```python
from build123d import *

# Parameters (mm, degrees)
BOSS_EXTRUDE1_DEPTH = 3
SKETCH2_R           = 1.5
SKETCH2_W           = 14
SKETCH2_H           = 7
CUT_EXTRUDE1_DEPTH  = 3


with BuildPart() as part:
    # Sketch1 → Boss-Extrude1 (new body)
    with BuildSketch(Plane(origin=(0, 0, 0), x_dir=(1, 0, 0), z_dir=(0, 1, 0))):
        Polygon((-41, -41), (-17.5, -41), (-17.5, -38), (17.5, -38), (17.5, -41), (41, -41), (41, -17.5), (38, -17.5), (38, 17.5), (41, 17.5), (41, 41), (17.5, 41), (17.5, 38), (-17.5, 38), (-17.5, 41), (-41, 41), (-41, 17.5), (-38, 17.5), (-38, -17.5), (-41, -17.5), align=None)
    extrude(amount=BOSS_EXTRUDE1_DEPTH)

    # Sketch2 → Cut-Extrude1 (cut)
    with BuildSketch(Plane(origin=(0, 3, 0), x_dir=(1, 0, 0), z_dir=(0, 1, 0))):
        with Locations((0, -8.5)):
            Circle(SKETCH2_R)
        with Locations((0, 13.5)):
            Rectangle(SKETCH2_W, SKETCH2_H)
    extrude(amount=-CUT_EXTRUDE1_DEPTH, mode=Mode.SUBTRACT)


solid = part.part
```
Input: part model. Units: mm. Frame: model coordinates. A direction names the side the tool comes from. Coordinates: 2 decimals unless noted, no trailing zeros. Loops run counter-clockwise (first coordinate to the right, second up) from the corner with the lowest first, then second, coordinate; pieces in that order, holes last.
Q1. Section D-D, the plane z = 8.5. Return the cut outline in (x, y).
Results are:
outline: (-38, 0) - (-1.5, 0) - (-1.5, 3) - (-38, 3) - close; (1.5, 0) - (38, 0) - (38, 3) - (1.5, 3) - close
Q2. Contact query for flat-ended pins moving along their axis: pin 1 (1.5 mm diameter, centred on y = 1, z = -13.5, fed in from +X); pin 2 (0.9 mm diameter, centred on x = -8.5, y = 1, fed in from +Z); pin 3 (0.9 mm diameter, centred on x = 0.5, y = 2, fed in from -Z). Output: stop coordinate, or through.
Results are:
pin 1: stops at x = 38
pin 2: stops at z = 38
pin 3: stops at z = -38
Q3. Section C-C, the plane y = 1.7. Return the cut outline in (x, z), and give its area (3 significant figures).
Results are:
outline: (-41, -41) - (-17.5, -41) - (-17.5, -38) - (17.5, -38) - (17.5, -41) - (41, -41) - (41, -17.5) - (38, -17.5) - (38, 17.5) - (41, 17.5) - (41, 41) - (17.5, 41) - (17.5, 38) - (-17.5, 38) - (-17.5, 41) - (-41, 41) - (-41, 17.5) - (-38, 17.5) - (-38, -17.5) - (-41, -17.5) - close; hole (-7, -17) - (7, -17) - (7, -10) - (-7, -10) - close; hole circle Ø3 at (0, 8.5)
area: 6,200 mm2
Q4. Section A-A, the plane x = 0. Return the cut outline in (y, z).
Results are:
outline: (0, -38) - (3, -38) - (3, -17) - (0, -17) - close; (0, -10) - (3, -10) - (3, 7) - (0, 7) - close; (0, 10) - (3, 10) - (3, 38) - (0, 38) - close
Q5. Line query: line 1 along Z through (x, y) = (0, 1); line 2 along X through (y, z) = (1.6, 8.5); line 3 along X through (y, z) = (0.7, -3.5). Output: solid intervals per line, ascending.
Results are:
line 1: z = -38 to -17, -10 to 7, 10 to 38
line 2: x = -38 to -1.5, 1.5 to 38
line 3: x = -38 to 38
Q6. Set-up query: faces 4 (the flat face through (39, 1, -17.5)), 5 (the flat face through (-17.5, 1, -39)), 6 (the flat face through (-38, 1, 0)), 7 (the flat face through (17.5, 1, 39)), 8 (the flat face through (0, 2, -17)). Return all of +Z, -Z, +X, -X, +Y, -Y with unobstructed straight access to the full face (end or side cutting, diameter ignored); none if empty.
Results are:
face 4: +X, +Y, -Y
face 5: -Z, +Y, -Y
face 6: -X, +Y, -Y
face 7: +Z, +Y, -Y
face 8: +Y, -Y
Q7. Section B-B, the plane z = -15.5. Return the cut outline in (x, y), and give its area (3 significant figures).
Results are:
outline: (-38, 0) - (-7, 0) - (-7, 3) - (-38, 3) - close; (7, 0) - (38, 0) - (38, 3) - (7, 3) - close
area: 186 mm2
Q8. Mould query, pull axis Z, two halves, no side actions, for faces 1 (the flat face through (0, 1, -38)), 2 (the flat face through (-1, 3, -1)), 3 (the cylindrical face through (0, 2, 10)). Classes: +Z half, -Z half, draft (parallel to the pull), parting line (faces both ways), or undercut.
Results are:
face 1: -Z half
face 2: draft
face 3: undercut
